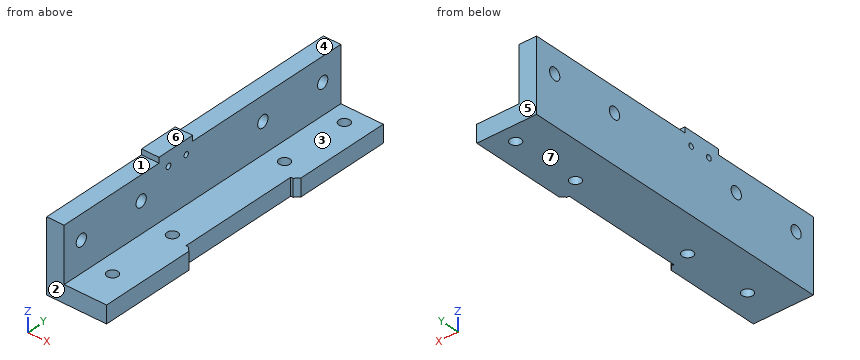
```python
from build123d import *

# Parameters (mm, degrees)
SKETCH1_W           = 24.51
SKETCH1_H           = 148
BOSS_EXTRUDE1_DEPTH = 8
SKETCH2_W           = 8
SKETCH2_H           = 148
BOSS_EXTRUDE2_DEPTH = 25
SKETCH3_R           = 2.5
CUT_EXTRUDE1_DEPTH  = 10
SKETCH4_R           = 2.75
CUT_EXTRUDE2_DEPTH  = 8
SKETCH5_W           = 3
SKETCH5_H           = 46
BOSS_EXTRUDE3_DEPTH = 8
SKETCH6_W           = 3
SKETCH6_H           = 46
BOSS_EXTRUDE4_DEPTH = 8
CHAMFER1_SIZE       = 2
SKETCH7_W           = 6
SKETCH7_H           = 18
BOSS_EXTRUDE5_DEPTH = 8
SKETCH8_R           = 1.175
SKETCH8_R_2         = 1.25
CUT_EXTRUDE3_DEPTH  = 8


with BuildPart() as part:
    # Sketch1 → Boss-Extrude1 (new body)
    with BuildSketch(Plane.XY):
        with Locations((-12.255, 74)):
            Rectangle(SKETCH1_W, SKETCH1_H)
    extrude(amount=BOSS_EXTRUDE1_DEPTH)

    # Sketch2 → Boss-Extrude2 (add)
    with BuildSketch(Plane.XY.offset(8)):
        with Locations((-20.51, 74)):
            Rectangle(SKETCH2_W, SKETCH2_H)
    extrude(amount=BOSS_EXTRUDE2_DEPTH)

    # Sketch3 → Cut-Extrude1 (cut)
    with BuildSketch(Plane.XY.offset(8)):
        with Locations((-8, 16)):
            Circle(SKETCH3_R)
        with Locations((-8, 48)):
            Circle(SKETCH3_R)
        with Locations((-8, 108)):
            Circle(SKETCH3_R)
        with Locations((-8, 140)):
            Circle(SKETCH3_R)
    extrude(amount=-CUT_EXTRUDE1_DEPTH, mode=Mode.SUBTRACT)

    # Sketch4 → Cut-Extrude2 (cut)
    with BuildSketch(Plane.ZY.offset(24.51)):
        with Locations((22, 138.3)):
            Circle(SKETCH4_R)
        with Locations((22, 106.3)):
            Circle(SKETCH4_R)
        with Locations((22, 41.2)):
            Circle(SKETCH4_R)
        with Locations((22, 9.2)):
            Circle(SKETCH4_R)
    extrude(amount=-CUT_EXTRUDE2_DEPTH, mode=Mode.SUBTRACT)

    # Sketch5 → Boss-Extrude3 (add)
    with BuildSketch(Plane(origin=(0, 0, 0), x_dir=(-1, 0, 0), z_dir=(0, 0, -1))):
        with Locations((-1.5, 125)):
            Rectangle(SKETCH5_W, SKETCH5_H)
    extrude(amount=-BOSS_EXTRUDE3_DEPTH)

    # Sketch6 → Boss-Extrude4 (add)
    with BuildSketch(Plane(origin=(0, 0, 0), x_dir=(-1, 0, 0), z_dir=(0, 0, -1))):
        with Locations((-1.5, 23)):
            Rectangle(SKETCH6_W, SKETCH6_H)
    extrude(amount=-BOSS_EXTRUDE4_DEPTH)

    # Chamfer1
    chamfer1_edges = [part.edges().sort_by_distance(p)[0] for p in [
        (3, 46, 4),
        (3, 102, 4),
    ]]
    chamfer(chamfer1_edges, length=CHAMFER1_SIZE)

    # Sketch7 → Boss-Extrude5 (add)
    with BuildSketch(Plane.ZY.offset(24.51)):
        with Locations((32.5, 59.722248883)):
            Rectangle(SKETCH7_W, SKETCH7_H)
    extrude(amount=-BOSS_EXTRUDE5_DEPTH)

    # Sketch8 → Cut-Extrude3 (cut)
    with BuildSketch(Plane.ZY.offset(24.51)):
        with Locations((29.112052986, 65.322248883)):
            Circle(SKETCH8_R)
        with Locations((29.112052986, 55.822248883)):
            Circle(SKETCH8_R_2)
    extrude(amount=-CUT_EXTRUDE3_DEPTH, mode=Mode.SUBTRACT)


solid = part.part
```
Input: part model. Units: mm. Frame: model coordinates. Face numbers are marked on the shaded views. A direction names the side the tool comes from. Round coordinates to 2 decimals unless told otherwise and drop trailing zeros. Loops run counter-clockwise (first coordinate to the right, second up) from the corner with the lowest first, then second, coordinate; pieces in that order, holes last. Notation, with made-up numbers: (-6, 83.5) - (3, 83.5) arc R12 ccw to (3, 102.5) - close; hole circle Ø6 at (46.5, 29.5). An arc over 180 degrees is marked (long way). One line per item, written item: value. Start each with the question number.
(1) Section B-B, the plane y = 48. Return loops of the section in (x, z), plus the area to 3 significant figures.
(2) Section C-C, the plane x = -8. Return loops of the section in (y, z), plus the area to 3 significant figures.
(3) Access query for the marked faces 1, 2, 3 and 4. Directions: +Z, -Z, +X, -X, +Y, -Y. A direction counts if a zero-diameter tool reaches every point of the face in a straight line with its end or side. Return the directions, or none.
(4) Section A-A, the plane z = 22. Return loops of the section in (x, y), plus the area to 3 significant figures.
(5) Draft query along Z for the marked faces 5, 6 and 7. Return one class per face: +Z half, -Z half, draft (parallel to the pull), parting line (faces both ways), or undercut.
(6) Contact query for flat-ended pins moving along their axis: P1, Ø4, axis at x = -14, y = 62.5, coming from the +Z side; P2, Ø12, axis at y = 19.5, z = 23.5, coming from the +X side; P3, Ø4.5, axis at x = -8, y = 140, coming from the -Z side; P4, Ø9, axis at x = -19.5, y = 124, coming from the +Z side. Output: stop coordinate, or through.
(7) Section D-D, the plane y = 23. Return loops of the section in (x, z), plus the area to 3 significant figures.
(8) Ray query, line 1 (Y direction, x = -8, z = 4.5); line 2 (X direction, y = 97.5, z = 7); line 3 (Z direction, x = -22.25, y = 112). Return the intervals inside material, ascending. Write a range as [from, to].
Results below:
1. outline: (-24.51, 0) - (-10.5, 0) - (-10.5, 8) - (-16.51, 8) - (-16.51, 33) - (-24.51, 33) - close; (-5.5, 0) - (0, 0) - (0, 8) - (-5.5, 8) - close
1. area: 356 mm^2
2. outline: (0, 0) - (13.5, 0) - (13.5, 8) - (0, 8) - close; (18.5, 0) - (45.5, 0) - (45.5, 8) - (18.5, 8) - close; (50.5, 0) - (105.5, 0) - (105.5, 8) - (50.5, 8) - close; (110.5, 0) - (137.5, 0) - (137.5, 8) - (110.5, 8) - close; (142.5, 0) - (148, 0) - (148, 8) - (142.5, 8) - close
2. area: 1,020 mm^2
3. face 1: +Z, +X, -X, -Y
3. face 2: +Z, -Z, +X, -X, -Y
3. face 3: +Z, +X, +Y, -Y
3. face 4: +Z, +X, -X, +Y
4. outline: (-24.51, 0) - (-16.51, 0) - (-16.51, 6.45) - (-24.51, 6.45) - close; (-24.51, 11.95) - (-16.51, 11.95) - (-16.51, 38.45) - (-24.51, 38.45) - close; (-24.51, 43.95) - (-16.51, 43.95) - (-16.51, 103.55) - (-24.51, 103.55) - close; (-24.51, 109.05) - (-16.51, 109.05) - (-16.51, 135.55) - (-24.51, 135.55) - close; (-24.51, 141.05) - (-16.51, 141.05) - (-16.51, 148) - (-24.51, 148) - close
4. area: 1,010 mm^2
5. face 5: draft
5. face 6: +Z half
5. face 7: -Z half
6. P1: z = 8
6. P2: x = -16.51
6. P3: through
6. P4: z = 33
7. outline: (-24.51, 0) - (3, 0) - (3, 8) - (-16.51, 8) - (-16.51, 33) - (-24.51, 33) - close
7. area: 420 mm^2
8. line 1: [0, 13.5], [18.5, 45.5], [50.5, 105.5], [110.5, 137.5], [142.5, 148]
8. line 2: [-24.51, 0]
8. line 3: [0, 33]
